from build123d import *

# Parameters (mm, degrees)
SKETCH_1_R               = 20
EXTRUDE_1_DEPTH          = 80
SKETCH_2_R               = 30
EXTRUDE_2_DEPTH          = 3
EXTRUDE_START            = 3
SKETCH_3_R               = 30
EXTRUDE_3_DEPTH          = 3
CUT_EXTRUDE_1_DEPTH      = 94.214805691
CUT_EXTRUDE_1_DEPTH_BACK = 94.214805691
SKETCH_4_R               = 1.25
FILLET_1_R               = 0.5
SKETCH_5_R               = 4
EXTRUDE_4_DEPTH          = 35
EXTRUDE_START_2          = 25
SKETCH_6_R               = 4
EXTRUDE_5_DEPTH          = 25
CHAMFER_4_SIZE           = 10
CHAMFER_5_SIZE           = 10


with BuildPart() as part:
    # 草图1 → 凸台-拉伸1 (new body)
    with BuildSketch(Plane(origin=(0, 0, 0), x_dir=(1, 0, 0), z_dir=(0, 1, 0))):
        with Locations(Location((0, 0, 0), (0, 0, 270))):
            Circle(SKETCH_1_R)
    extrude(amount=EXTRUDE_1_DEPTH)

    # 草图2 → 凸台-拉伸2 (add)
    with BuildSketch(Plane(origin=(0, 80, 0), x_dir=(1, 0, 0), z_dir=(0, 1, 0))):
        with Locations(Location((0, 0, 0), (0, 0, 270))):
            Circle(SKETCH_2_R)
    extrude(amount=EXTRUDE_2_DEPTH)

    # 草图3 → 凸台-拉伸3 (add)
    with BuildSketch(Plane.XZ.offset(EXTRUDE_START)):
        with Locations(Location((0, 0, 0), (0, 0, 90))):
            Circle(SKETCH_3_R)
    extrude(amount=-EXTRUDE_3_DEPTH)

    # 草图4 → 切除-拉伸1 (cut, two sides: drawn at the far end of the back side and taken through both)
    with BuildSketch(Plane.XY.offset(-CUT_EXTRUDE_1_DEPTH_BACK)):
        with Locations((17, 26.5)):
            Circle(SKETCH_4_R)
    extrude(amount=CUT_EXTRUDE_1_DEPTH + CUT_EXTRUDE_1_DEPTH_BACK, mode=Mode.SUBTRACT)

    # 圆角1
    fillet_1_edges = [part.edges().sort_by_distance(p)[0] for p in [
        (0, 0, -30),
        (0, -3, -30),
        (0, 80, -30),
        (0, 83, -30),
    ]]
    fillet(fillet_1_edges, radius=FILLET_1_R)

    # 草图5 → 凸台-拉伸4 (add)
    with BuildSketch(Plane(origin=(0, 83, 0), x_dir=(1, 0, 0), z_dir=(0, 1, 0))):
        with Locations(Location((0, 0, 0), (0, 0, 270))):
            Circle(SKETCH_5_R)
    extrude(amount=EXTRUDE_4_DEPTH)

    # 草图6 → 凸台-拉伸5 (add)
    with BuildSketch(Plane(origin=(0, -3, 0), x_dir=(-1, 0, 0), z_dir=(0, -1, 0)).offset(EXTRUDE_START_2)):
        with Locations(Location((0, 0, 0), (0, 0, 270))):
            Circle(SKETCH_6_R)
    extrude(amount=-EXTRUDE_5_DEPTH)

    # 倒角4
    chamfer_4_edges = [part.edges().sort_by_distance(p)[0] for p in [
        (0, 83, -4),
    ]]
    chamfer(chamfer_4_edges, length=CHAMFER_4_SIZE)

    # 倒角5
    chamfer_5_edges = [part.edges().sort_by_distance(p)[0] for p in [
        (0, -3, -4),
    ]]
    chamfer(chamfer_5_edges, length=CHAMFER_5_SIZE)


solid = part.part
Could you check a few things on this model? Use its own coordinates, in mm. A direction names the side the tool comes from. Give positions to 0.01 mm unless a question says otherwise; leave off trailing zeros. Write each loop counter-clockwise with the first axis right and the second up, starting at its lowest first coordinate (ties: lowest second). Pieces come first, ordered by that corner, then holes. Notation, with made-up numbers: (28.25, -14.75) - (63.25, -14.75) arc R17 ccw to (63.25, 10.25) - close; hole circle Ø6 at (-31.5, -33). An arc over 180 degrees is marked (long way). Use CSV: the item, a comma, the result in double quotes. Start each with the question number.
Item 1: For faces 1 (the face through (-6, 83, 13)), 2 (the face through (-19.524, 39.44, -4.336)), 3 (the face through (6, -3, 13)), which set-ups out of +Z, -Z, +X, -X, +Y, -Y let a thin tool reach every point of the face, with its end or its side?
Item 2: If I drill on line 1 along Y through (x, z) = (4, 24); line 2 along Y through (x, z) = (17, -2); line 3 along X through (y, z) = (26.5, -1), over which ranges is the centre line in solid material (lowest first)?
Item 3: If we mould it in two halves opening along Y, with no side actions, what happens to faces 4 (the face through (-19.3, 80, 6.1)), 5 (the face through (-4.45, -12.51, -0.58)), 6 (the face through (0, 118, 0))? For each: pulls with the +Y half, pulls with the -Y half, needs draft (parallel to the pull), parting line crosses it, or undercut.
Item 4: I'm going to push flat-ended pins straight in: pin 1 (1 mm diameter, centred on x = -17, y = 36, fed in from +Z); pin 2 (1.5 mm diameter, centred on y = 83, z = 17.5, fed in from +X); pin 3 (4 mm diameter, centred on x = -15, z = 4, fed in from +Y). Where does each tip first touch, or does it pass through?
Item 5: I want a section at D-D, the plane y = 85. Please give me the cut outline in (x, z).
Item 6: I want a section at C-C, the plane y = 100.5. Please give me the cut outline in (x, z), then the cut area to 3 significant figures.
Findings:
1,face 1,"+Y"
1,face 2,"none"
1,face 3,"-Y"
2,line 1,"y = -3 to 0, 80 to 83"
2,line 2,"y = -3 to 25.25, 27.75 to 83"
2,line 3,"x = -19.97 to 15.75, 18.25 to 19.97"
3,face 4,"undercut"
3,face 5,"pulls with the -Y half"
3,face 6,"pulls with the +Y half"
4,pin 1,"stops at z = 11.3"
4,pin 2,"stops at x = 24.8"
4,pin 3,"stops at y = 83.48"
5,outline,"circle Ø24 at (0, 0)"
6,outline,"circle Ø8 at (0, 0)"
6,area,"50.3 mm2"
